Verification items for the finished model (mm, model axes). Round coordinates to 2 decimals unless told otherwise and drop trailing zeros. Loops run counter-clockwise (first coordinate to the right, second up) from the corner with the lowest first, then second, coordinate; pieces in that order, holes last. Notation, with made-up numbers: M 10,-3 L 35,-3 A26 ccw 35,17 Z; hole C -3,8 d8. An arc over 180 degrees is marked long. One line per item, written item: value.
from build123d import *

# Parameters (mm, degrees)
BOSS_EXTRUDE1_DEPTH = 3.175
FILLET1_R           = 6.35
SKETCH2_R           = 3.302
CUT_EXTRUDE1_DEPTH  = 161.944735796
SKETCH3_R           = 2.54
SKETCH3_R_2         = 2.032
CUT_EXTRUDE2_DEPTH  = 161.944735796
SKETCH4_R           = 14.2875
SKETCH4_R_2         = 11.176
SKETCH4_R_3         = 2.54
SKETCH4_R_4         = 2.032
CUT_EXTRUDE3_DEPTH  = 161.944735796
SKETCH5_R           = 4.826
CUT_EXTRUDE4_DEPTH  = 161.944735796
BOSS_EXTRUDE2_DEPTH = 3.175
FILLET2_R           = 12.7
FILLET3_R           = 12.7


with BuildPart() as part:
    # Sketch1 → Boss-Extrude1 (new body)
    with BuildSketch(Plane.XY):
        Polygon((0, 0), (-82.55, 0), (-107.95, -120.65), (25.4, -120.65), align=None)
    extrude(amount=BOSS_EXTRUDE1_DEPTH)

    # Fillet1
    fillet1_edges = [part.edges().sort_by_distance(p)[0] for p in [
        (25.4, -120.65, 1.5875),
        (-107.95, -120.65, 1.5875),
        (-82.55, 0, 1.5875),
        (0, 0, 1.5875),
    ]]
    fillet(fillet1_edges, radius=FILLET1_R)

    # Sketch2 → Cut-Extrude1 (cut, through all)
    with BuildSketch(Plane(origin=(0, 0, 0), x_dir=(-1, 0, 0), z_dir=(0, 0, -1))):
        with Locations((-14.2875, -114.3)):
            Circle(SKETCH2_R)
        with Locations((96.8375, -114.3)):
            Circle(SKETCH2_R)
    extrude(amount=-CUT_EXTRUDE1_DEPTH, mode=Mode.SUBTRACT)

    # Sketch3 → Cut-Extrude2 (cut, through all)
    with BuildSketch(Plane(origin=(0, 0, 0), x_dir=(-1, 0, 0), z_dir=(0, 0, -1))):
        with Locations((9.525, -13.462)):
            Circle(SKETCH3_R)
        with Locations((73.025, -13.462)):
            Circle(SKETCH3_R)
        with Locations((3.683, -13.462)):
            Circle(SKETCH3_R_2)
        with Locations((78.867, -13.462)):
            Circle(SKETCH3_R_2)
    extrude(amount=-CUT_EXTRUDE2_DEPTH, mode=Mode.SUBTRACT)

    # Sketch4 → Cut-Extrude3 (cut, through all)
    with BuildSketch(Plane.XY.offset(3.175)):
        with Locations((-41.275, -84.074)):
            Circle(SKETCH4_R)
        with Locations((-41.275, -43.434)):
            Circle(SKETCH4_R_2)
        with Locations((-2.667, -102.616)):
            Circle(SKETCH4_R_3)
        with Locations((-79.883, -102.616)):
            Circle(SKETCH4_R_3)
        with Locations((-85.725, -102.616)):
            Circle(SKETCH4_R_4)
        with Locations((3.175, -102.616)):
            Circle(SKETCH4_R_4)
    extrude(amount=-CUT_EXTRUDE3_DEPTH, mode=Mode.SUBTRACT)

    # Sketch5 → Cut-Extrude4 (cut, through all)
    with BuildSketch(Plane.XY.offset(3.175)):
        with Locations((-80.01, -30.48)):
            Circle(SKETCH5_R)
        with Locations((-80.01, -55.88)):
            Circle(SKETCH5_R)
        with Locations((-80.01, -81.28)):
            Circle(SKETCH5_R)
        with Locations((-2.54, -81.28)):
            Circle(SKETCH5_R)
        with Locations((-2.54, -55.88)):
            Circle(SKETCH5_R)
        with Locations((-2.54, -30.48)):
            Circle(SKETCH5_R)
    extrude(amount=-CUT_EXTRUDE4_DEPTH, mode=Mode.SUBTRACT)

    # Sketch6 → Boss-Extrude2 (add)
    with BuildSketch(Plane.XY.offset(3.175)):
        with BuildLine():
            Line((-88.378631579, -27.686), (-168.275, -27.686))
            Line((-168.275, -27.686), (-168.275, 175.514))
            Line((-168.275, 175.514), (85.725, 175.514))
            Line((85.725, 175.514), (85.725, -27.686))
            Line((85.725, -27.686), (5.828631579, -27.686))
            Line((5.828631579, -27.686), (1.06143862, -5.041833445))
            ThreePointArc((1.06143862, -5.041833445), (-1.151374985, -1.419008334), (-5.152352515, 0))
            Line((-5.152352515, 0), (-77.397647485, 0))
            ThreePointArc((-77.397647485, 0), (-81.398625015, -1.419008334), (-83.61143862, -5.041833445))
            Line((-83.61143862, -5.041833445), (-88.378631579, -27.686))
        make_face()
    extrude(amount=-BOSS_EXTRUDE2_DEPTH)

    # Fillet2
    fillet2_edges = [part.edges().sort_by_distance(p)[0] for p in [
        (-88.378631579, -27.686, 1.5875),
        (5.828631579, -27.686, 1.5875),
    ]]
    fillet(fillet2_edges, radius=FILLET2_R)

    # Fillet3
    fillet3_edges = [part.edges().sort_by_distance(p)[0] for p in [
        (-168.275, -27.686, 1.5875),
        (-168.275, 175.514, 1.5875),
        (85.725, 175.514, 1.5875),
        (85.725, -27.686, 1.5875),
    ]]
    fillet(fillet3_edges, radius=FILLET3_R)


solid = part.part
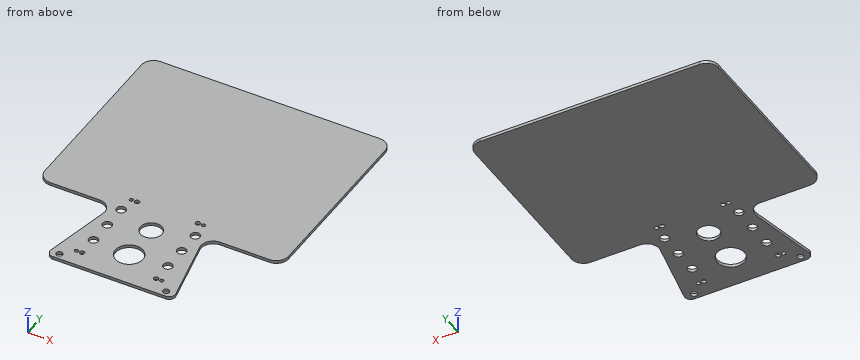
(1) Sectioned sample at A-A on z = 2.5. Count the separate pieces of the cut face and the enclosed holes in it, and give its area (3 significant figures).
Completed:
separate pieces: 1
enclosed holes: 18
area: 60,500 mm^2
(2) Sectioned sample at B-B on x = -148. Enter the section's corners in (y, z) (3 decimals).
Completed:
outline: M -27.686,0 L 175.514,0 L 175.514,3.175 L -27.686,3.175 Z
(3) Depth check by flat-ended pin: pin 1 Ø1.6 at (x, z) = (46, 2) entering from -Y. Enter the tip coordinate at first touch or a pass-through.
Completed:
pin 1: stops at y = -27.69
(4) Thickness scan on L1, parallel to Y at x = -41.5, z = 0.15; L2, parallel to X at y = -84.5, z = 1.6; L3, parallel to Y at x = -80.01, z = 1. Record the ranges inside material, lowest first. Write a range as from..to.
Completed:
L1: y = -120.65..-98.36, -69.79..-54.61, -32.26..175.51
L2: x = -100.34..-83.6, -76.42..-55.56, -26.99..-6.13, 1.05..17.79
L3: y = -120.65..-105.15, -100.08..-86.11, -76.45..-60.71, -51.05..-35.31, -25.65..-15.14, -11.78..175.51
